from build123d import *

# Parameters (mm, degrees)
F1_DEPTH  = 14.224
F2_W      = 104.648
F2_H      = 28.575
F3_DEPTH  = 7.874
F5_DEPTH  = 4.826
F6_W      = 28.702
F6_H      = 17.526
F7_DEPTH  = 12.7
F9_DEPTH  = 12.7
F11_DEPTH = 25.4


with BuildPart() as f1:
    # F0 (on Front) → F1 (new body, symmetric)
    with BuildSketch(Plane.XZ):
        Polygon((32.3041829584, 0.0577278724), (32.3041829584, 15.9327278724), (-41.1018170416, 15.9327278724), (-41.1018170416, 0), align=None)
    extrude(amount=F1_DEPTH, both=True)

    # F2 (on Front) → F3 (join, symmetric)
    with BuildSketch(Plane.XZ):
        with Locations((11.0836382955, 30.133637134)):
            Rectangle(F2_W, F2_H)
    extrude(amount=F3_DEPTH, both=True)

    # F4 (on face) → F5 (cut)
    with BuildSketch(Plane.XZ.offset(7.874)):
        Polygon((-34.8903617045, 44.421137134), (-41.2403617045, 44.421137134), (-41.2403617045, 15.846137134), (-41.1018170416, 15.846137134), (-41.1018170416, 15.9327278724), (-34.8903617045, 15.9327278724), align=None)
    extrude(amount=-F5_DEPTH, mode=Mode.SUBTRACT)

    # F6 (on Front) → F7 (join, symmetric)
    with BuildSketch(Plane.XZ):
        with Locations((49.0566382955, 35.658137134)):
            Rectangle(F6_W, F6_H)
    extrude(amount=F7_DEPTH, both=True)

    # F8 (on Front) → F9 (cut, symmetric)
    with BuildSketch(Plane.XZ):
        Polygon((63.4076382955, 44.421137134), (34.0538099408, 15.824187547), (63.4076382955, 15.846137134), align=None)
    extrude(amount=F9_DEPTH, both=True, mode=Mode.SUBTRACT)

    # F10 (on face) → F11 (cut)
    with BuildSketch(Plane.XZ.offset(7.874)):
        with BuildLine():
            ThreePointArc((13.0001829584, 35.7447278724), (7.4121829584, 30.1567278724), (13.0001829584, 24.5687278724))
            ThreePointArc((13.0001829584, 24.5687278724), (16.9514956516, 26.2054151791), (18.5881829584, 30.1567278724))
            ThreePointArc((18.5881829584, 30.1567278724), (16.9514956516, 34.1080405657), (13.0001829584, 35.7447278724))
        make_face()
        with BuildLine():
            ThreePointArc((-10.8758170416, 35.7447278724), (-16.4638170416, 30.1567278724), (-10.8758170416, 24.5687278724))
            ThreePointArc((-10.8758170416, 24.5687278724), (-6.9245043484, 26.2054151791), (-5.2878170416, 30.1567278724))
            ThreePointArc((-5.2878170416, 30.1567278724), (-6.9245043484, 34.1080405657), (-10.8758170416, 35.7447278724))
        make_face()
        with BuildLine():
            ThreePointArc((-5.2878170416, 30.1567278724), (-6.9245043484, 26.2054151791), (-10.8758170416, 24.5687278724))
            Line((-10.8758170416, 24.5687278724), (13.0001829584, 24.5687278724))
            ThreePointArc((13.0001829584, 24.5687278724), (7.4121829584, 30.1567278724), (13.0001829584, 35.7447278724))
            Line((13.0001829584, 35.7447278724), (-10.8758170416, 35.7447278724))
            ThreePointArc((-10.8758170416, 35.7447278724), (-6.9245043484, 34.1080405657), (-5.2878170416, 30.1567278724))
        make_face()
    extrude(amount=-F11_DEPTH, mode=Mode.SUBTRACT)

    # F12: F1 across face


with BuildPart() as f1_1:
    add(f1.part)
    add(f1.part.mirror(Plane(origin=(-4.3988170416, 0, 0.0288639362), x_dir=(1, 0, 0), z_dir=(0.0007864187, 0, -0.9999996908))))


solid = f1_1.part
Input: part model. Units: mm. Frame: model coordinates. A direction names the side the tool comes from. Coordinates: 2 decimals unless noted, no trailing zeros. Write each loop counter-clockwise with the first axis right and the second up, starting at its lowest first coordinate (ties: lowest second). Pieces come first, ordered by that corner, then holes. Notation, with made-up numbers: M -37.75,41.5 L -30.75,41.5 A14 ccw -30.75,55.5 Z; hole C -32.5,1.5 d11. An arc over 180 degrees is marked long. Answer as a JSON object with one key per item and string values. Group by question number.
(1) Section D-D on x = 47. Output: boundary loops of the cut face in (y, z), plus the area to 3 significant figures.
(2) Contact query for flat-ended pins moving along their axis: P1, Ø9, axis at x = 55, z = -31.5, coming from the -Y side; P2, Ø4, axis at x = -17, y = 2, coming from the -Z side; P3, Ø7, axis at x = -38.5, z = -37, coming from the -Y side. Output: stop coordinate, or through.
(3) Section A-A on y = -9.25. Output: boundary loops of the cut face in (x, z).
(4) Section C-C on y = 4. Output: boundary loops of the cut face in (x, z), plus the area to 3 significant figures.
(5) Ray query, line 1 along Z through (x, y) = (-5, -6.25); line 2 along X through (y, z) = (-7.75, -6); line 3 along Z through (x, y) = (50, 2.5). Return the intervals inside material, ascending. Write a range as [from, to].
(6) Mould query, pull axis X, two halves, no side actions, for faces 4 (the face through (1, 0, 24.569)), 5 (the face through (-34.89, -5, 30)), 6 (the face through (5, -7.874, 24)). Classes: pulls with the +X half, pulls with the -X half, needs draft (parallel to the pull), parting line crosses it, or undercut.
(7) Set-up query: faces 1 (the face through (52.2, -0.2, 33.5)), 2 (the face through (40, 10, 26.895)), 3 (the face through (-5, 14.224, 0)). Return all of +Z, -Z, +X, -X, +Y, -Y with unobstructed straight access to the full face (end or side cutting, diameter ignored); none if empty.
(8) Section B-B on x = 3. Output: boundary loops of the cut face in (y, z).
Result set:
{
 "1": {"outline": "M -12.7,-44.28 L 12.7,-44.28 L 12.7,-28.25 L -12.7,-28.25 Z; M -12.7,28.44 L 12.7,28.44 L 12.7,44.42 L -12.7,44.42 Z", "area": "813 mm2"},
 "2": {"P1": "stops at y = -12.7", "P2": "stops at z = -44.39", "P3": "stops at y = -3.05"},
 "3": {"outline": "M -41.1,0 L -41.08,-15.93 L 32.33,-15.82 L 32.3,0.06 L 32.3,15.93 L -41.1,15.93 Z; M 34.71,26.9 L 45.42,26.9 L 63.41,44.42 L 34.71,44.42 Z; M 34.75,-26.78 L 34.78,-44.3 L 63.48,-44.26 L 45.46,-26.76 Z"},
 "4": {"outline": "M -41.24,15.85 L -41.1,15.85 L -41.1,0 L -41.08,-15.85 L -41.22,-15.85 L -41.17,-44.42 L 63.48,-44.26 L 34.1,-15.73 L 32.33,-15.73 L 32.3,0.06 L 32.3,15.85 L 34.08,15.85 L 63.41,44.42 L -41.24,44.42 Z; hole M -10.88,24.57 L 13,24.57 A5.59 ccw 13,35.74 L -10.88,35.74 A5.59 ccw Z; hole M -10.84,-24.52 A5.59 ccw -10.82,-35.7 L 13.06,-35.66 A5.59 ccw 13.04,-24.48 Z", "area": "6,730 mm2"},
 "5": {"line 1": "z = [-44.36, -35.69], [-24.51, 24.57], [35.74, 44.42]", "line 2": "x = [-41.09, 32.31]", "line 3": "z = [-44.28, -31.17], [31.36, 44.42]"},
 "6": {"face 4": "undercut", "face 5": "pulls with the -X half", "face 6": "needs draft"},
 "7": {"face 1": "+X, +Y, -Y", "face 2": "+X, -X, +Y", "face 3": "+Z, -Z, +X, -X, +Y"},
 "8": {"outline": "M -14.22,-15.86 L -7.87,-15.86 L -7.87,-24.5 L 7.87,-24.5 L 7.87,-15.86 L 14.22,-15.86 L 14.22,15.93 L 7.87,15.93 L 7.87,24.57 L -7.87,24.57 L -7.87,15.93 L -14.22,15.93 Z; M -7.87,-44.35 L 7.87,-44.35 L 7.87,-35.68 L -7.87,-35.68 Z; M -7.87,35.74 L 7.87,35.74 L 7.87,44.42 L -7.87,44.42 Z"}
}
